Source: CAD feature listing. Evaluate the final solid. Frame: model axes, mm. Face numbers are marked on the shaded views. A direction names the side the tool comes from. Round coordinates to 2 decimals unless told otherwise and drop trailing zeros. Write each loop counter-clockwise with the first axis right and the second up, starting at its lowest first coordinate (ties: lowest second). Pieces come first, ordered by that corner, then holes. Notation, with made-up numbers: M 14.5,58 L 61.5,58 A10 cw 61.5,62 Z; hole C 32.5,59 d6. An arc over 180 degrees is marked long. Use a Markdown table: item, result.
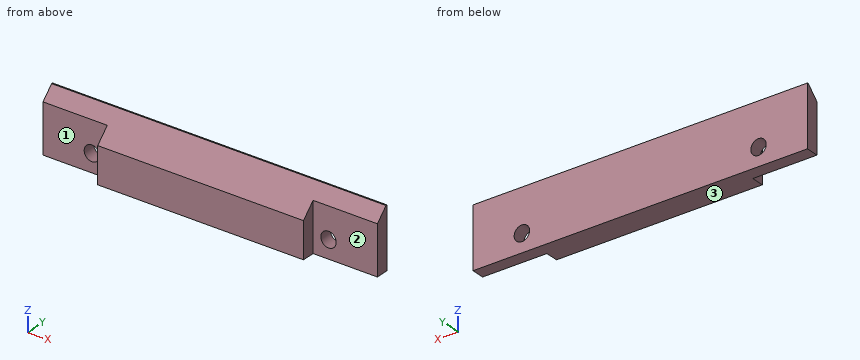
Autodesk Inventor part; units mm, degrees
ref_plane "YZ Plane" through (0, 0, 0) normal (1, 0, 0) x (0, 1, 0)
ref_plane "XZ Plane" through (0, 0, 0) normal (0, 1, 0) x (-1, 0, 0)
ref_plane "XY Plane" through (0, 0, 0) normal (0, 0, 1) x (1, 0, 0)
sketch "Sketch1" plane through (0, 0, 0) normal (1, 0, 0) x (0, 1, 0)
  line L0 (0, 0) -> (0, -36)
  line L1 (0, -36) -> (-5, -36)
  line L2 (-5, -36) -> (-5, -5)
  line L3 (-5, -5) -> (0, 0)
  dimension "d1" = 5
  dimension "d2" = 45
  dimension "d5" = 31
extrude "Extrusion1" add sketch "Sketch1" along normal blind 130
sketch "Sketch2" plane through (130, 0, 0) normal (1, 0, 0) x (0, 0, -1)
  line L0 (36, 0) -> (0, 0)
  line L1 (0, 0) -> (0.5, 0)
  line L2 (0.5, 0) -> (0.5, -0.5)
  line L3 (0, 0) -> (5, -5)
  line L4 (0, 0) -> (0.5, -0.5)
  dimension "d6" = 0.5
extrude "Extrusion2" cut sketch "Sketch2" against normal through all
sketch "Sketch3" plane through (0, 0, -36) normal (0, 1, 0) x (1, 0, 0)
  circle A0 centre (19, -6) radius 3
  circle A1 centre (19, -19) radius 3
  line L0 (0, -35.5) -> (0, 0)
  line L1 (0, 0) -> (130, 0)
  circle A2 centre (111, -6) radius 3
  circle A3 centre (111, -19) radius 3
  line L2 (130, 0) -> (130, -35.5)
  point P0 (0, -36)
  dimension "d9" = 6
  dimension "d10" = 6
  dimension "d11" = 19
  dimension "d12" = 13
  dimension "d13" = 6
  dimension "d16" = 6
  dimension "d17" = 6
  dimension "d18" = 19
  dimension "d19" = 13
extrude "Extrusion4" cut sketch "Sketch3" against normal up to next
sketch "Sketch4" plane through (0, -5, -36) normal (0, -1, 0) x (1, 0, 0)
  line L0 (0, 0) -> (130, 0)
  line L1 (0, 31) -> (130, 31)
  line L2 (25, 0) -> (105, 0)
  line L3 (105, 0) -> (105, 31)
  line L4 (105, 31) -> (25, 31)
  line L5 (25, 31) -> (25, 0)
  line L6 (130, 31) -> (130, 0)
  point P0 (0, 36)
  dimension "d22" = 25
  dimension "d23" = 25
extrude "Extrusion5" add sketch "Sketch4" along normal blind 5 contours L5 L1 L3 L0
sketch "Sketch5" plane through (25, -5, -36) normal (-1, 0, 0) x (0, 0, 1)
  line L0 (31, 0) -> (31, -5)
  line L1 (31, 0) -> (31, -5)
  line L2 (31, -5) -> (26, -5)
  line L3 (0, -5) -> (31, -5)
  line L4 (26, -5) -> (31, 0)
  point P0 (36, 5)
  dimension "d26" = 5
extrude "Extrusion6" cut sketch "Sketch5" against normal up to next
sketch "Sketch6" plane through (130, 0, 0) normal (1, 0, 0) x (0, 0, -1)
  line L0 (0.5, 0) -> (0.5, -0.5)
  line L1 (0.5, -0.5) -> (5, -5)
  line L2 (5, -5) -> (36, -5)
  line L3 (36, -5) -> (36, 0)
  line L4 (36, 0) -> (0.5, 0)
  line L5 (5, -5) -> (10, -10)
  line L6 (36, -10) -> (10, -10)
  line L7 (36, -5) -> (36, -10)
  line L8 (5, -5) -> (36, -5)
  line L9 (36, 0) -> (24, 0)
  line L10 (24, 0) -> (24, -5)
  line L11 (24, -5) -> (36, -5)
  line L12 (36, -5) -> (36, 0)
  point P0 (0, 0)
  dimension "d29" = 12
  dimension "d30" = 5
extrude "Extrusion7" cut sketch "Sketch6" against normal through all contours L4 L3 L2 L10
sketch "Sketch7" plane through (105, -10, -10) normal (1, 0, 0) x (0, 0, -1)
  line L0 (-5, 5) -> (0, 0)
  line L1 (26, 0) -> (0, 0)
  line L2 (26, 5) -> (26, 0)
  line L3 (14, 5) -> (26, 5)
  line L4 (-5, 5) -> (14, 5)
  line L5 (14, 5) -> (14, 10)
  line L6 (14, 10) -> (-9.5, 10)
  line L7 (-9.5, 10) -> (-9.5, 9.5)
  line L8 (-9.5, 9.5) -> (-5, 5)
  line L9 (-5, 5) -> (14, 5)
  line L10 (26, 0) -> (14, 0)
  line L11 (14, 0) -> (14, 5)
  line L12 (14, 5) -> (26, 5)
  line L13 (26, 5) -> (26, 0)
  point P0 (-10, 10)
extrude "Extrusion8" cut sketch "Sketch7" against normal through all contours L3 L2 L1 L11
properties part number "back_beam"
Q1. Reachability of the marked faces 1, 2 and 3 from +Z, -Z, +X, -X, +Y, -Y: full face, straight path, thin tool, end or side. Return the list, or none.
Results are:
| item | result |
|---|---|
| face 1 | +Z, -Z, -X, -Y |
| face 2 | +Z, -Z, +X, -Y |
| face 3 | -Z, +X, -X, +Y, -Y |
Q2. Section B-B on z = -17. Return loops of the section in (x, y).
Results are:
| item | result |
|---|---|
| outline | M 0,-5 L 16,-5 L 16,0 L 0,0 Z; M 22,-5 L 25,-5 L 25,-10 L 105,-10 L 105,-5 L 108,-5 L 108,0 L 22,0 Z; M 114,-5 L 130,-5 L 130,0 L 114,0 Z |
Q3. First-contact query: pin 1 Ø2.5 at (y, z) = (-7, -14) entering from -X; pin 2 Ø1 at (x, y) = (84.5, -8.5) entering from +Z; pin 3 Ø1.5 at (y, z) = (-7.5, -13.5) entering from +X; pin 4 Ø5.5 at (x, z) = (111, -17) entering from -Y. Flat tips, straight axial feed; report the tip coordinate or a pass-through.
Results are:
| item | result |
|---|---|
| pin 1 | x = 25 |
| pin 2 | z = -8 |
| pin 3 | x = 105 |
| pin 4 | through |
Q4. Section C-C on y = -2.75. Return loops of the section in (x, z).
Results are:
| item | result |
|---|---|
| outline | M 0,-24 L 130,-24 L 130,-2.75 L 0,-2.75 Z; hole C 19,-17 d6; hole C 111,-17 d6 |
Q5. Line query: L1, parallel to X at y = -3.3, z = -17; L2, parallel to Y at x = 114, z = -9.75; L3, parallel to X at y = -7, z = -18.5. Output: solid intervals per line, ascending.
Results are:
| item | result |
|---|---|
| L1 | 0 to 16, 22 to 108, 114 to 130 |
| L2 | -5 to 0 |
| L3 | 25 to 105 |
Q6. Section A-A on x = 111. Return loops of the section in (y, z), plus the area to 3 significant figures.
Results are:
| item | result |
|---|---|
| outline | M -5,-24 L 0,-24 L 0,-20 L -5,-20 Z; M -5,-14 L 0,-14 L 0,-0.5 L -0.5,-0.5 L -5,-5 Z |
| area | 77.4 mm^2 |
Q7. Section D-D on z = -12. Return loops of the section in (x, y), plus the area to 3 significant figures.
Results are:
| item | result |
|---|---|
| outline | M 0,-5 L 25,-5 L 25,-10 L 105,-10 L 105,-5 L 130,-5 L 130,0 L 0,0 Z |
| area | 1,050 mm^2 |
